Source: three-view drawing plus pictorial views. Frame: mm from the lowest corner of the part. A direction names the side the tool comes from. Coordinates: 2 decimals unless noted, no trailing zeros. Write each loop counter-clockwise with the first axis right and the second up, starting at its lowest first coordinate (ties: lowest second). Pieces come first, ordered by that corner, then holes. Notation, with made-up numbers: M 14.5,-25.75 L 71.5,-25.75 A17 cw 71.5,-10.75 Z; hole C -14,43 d2. An arc over 180 degrees is marked long. Answer as a JSON object with one key per item and string values. Group by question number.
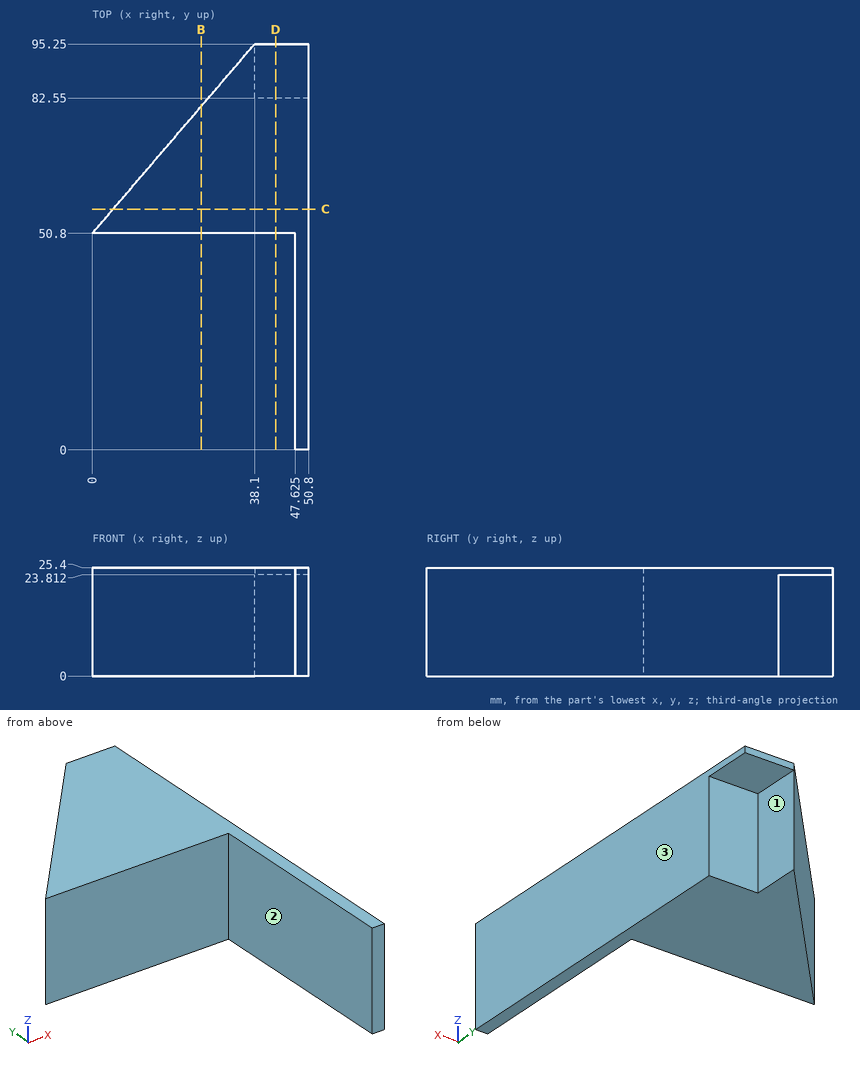
Q1. Pin query (flat end, axial travel): pin 1 Ø10 at (y, z) = (86.5, 12) entering from +X; pin 2 Ø12.5 at (y, z) = (16, 7) entering from -X (1 decimal); pin 3 Ø2 at (x, z) = (14.5, 5) entering from -Y; pin 4 Ø10 at (x, z) = (47, 11.5) entering from +Y. Return the tip coordinate at first contact, or that it passes through.
Q2. Section B-B, the plane x = 25.5. Return the cut outline in (y, z), and give its area (3 significant figures).
Q3. Access query for the marked faces 1, 2 and 3. Directions: +Z, -Z, +X, -X, +Y, -Y. A direction counts if a zero-diameter tool reaches every point of the face in a straight line with its end or side. Return the directions, or none.
Q4. Section D-D, the plane x = 43. Return the cut outline in (y, z).
Q5. Section C-C, the plane y = 56.5. Return the cut outline in (x, z) (1 decimal), and give its area (3 significant figures).
Q6. Line query: line 1 (X direction, y = 12, z = 3) (1 decimal); line 2 (Y direction, x = 46, z = 7.75); line 3 (Y direction, x = 13.5, z = 3.5). Output: solid intervals per line, ascending. Write a range as from..to.
Filled in:
{
 "1": {"pin 1": "x = 50.8", "pin 2": "x = 47.6", "pin 3": "y = 50.8", "pin 4": "y = 82.55"},
 "2": {"outline": "M 50.8,0 L 80.55,0 L 80.55,25.4 L 50.8,25.4 Z", "area": "756 mm^2"},
 "3": {"face 1": "-Z, +X, +Y", "face 2": "+Z, -Z, -X, -Y", "face 3": "+Z, -Z, +X, +Y, -Y"},
 "4": {"outline": "M 50.8,0 L 82.55,0 L 82.55,23.81 L 95.25,23.81 L 95.25,25.4 L 50.8,25.4 Z"},
 "5": {"outline": "M 4.9,0 L 50.8,0 L 50.8,25.4 L 4.9,25.4 Z", "area": "1,170 mm^2"},
 "6": {"line 1": "47.6..50.8", "line 2": "50.8..82.55", "line 3": "50.8..66.55"}
}
